```python
from build123d import *

# Parameters (mm, degrees)
SKIZZE2_W                        = 120
SKIZZE2_H                        = 39.364160046
AUFSATZ_LINEAR_AUSTRAGEN1_DEPTH  = 30
SKIZZE24_R                       = 1.55
SCHNITT_LINEAR_AUSTRAGEN4_DEPTH  = 130.805766806
SKIZZE46_R                       = 2.85
SCHNITT_LINEAR_AUSTRAGEN15_DEPTH = 10
SCHNITT_LINEAR_START             = -5
SCHNITT_LINEAR_AUSTRAGEN25_DEPTH = 2.7
LINEARES_MUSTER1_COUNT           = 5
LINEARES_MUSTER1_PITCH           = 20
SPIEGELN2_COPY_1_SKETCH_R        = 2.85
SPIEGELN2_COPY_1_DEPTH           = 10
SPIEGELN2_COPY_2_SKETCH_R        = 2.85
SPIEGELN2_COPY_2_DEPTH           = 10
SPIEGELN2_COPY_3_SKETCH_R        = 2.85
SPIEGELN2_COPY_3_DEPTH           = 10
SPIEGELN2_COPY_4_SKETCH_R        = 2.85
SPIEGELN2_COPY_4_DEPTH           = 10
SPIEGELN2_START                  = -5
SPIEGELN2_COPY_5_DEPTH           = 2.7
SPIEGELN2_COPY_6_DEPTH           = 2.7
SPIEGELN2_COPY_7_DEPTH           = 2.7
SPIEGELN2_COPY_8_DEPTH           = 2.7
SKIZZE51_R                       = 1.55
SCHNITT_LINEAR_AUSTRAGEN26_DEPTH = 130.805766806
SKIZZE67_R                       = 0.5
SCHNITT_LINEAR_AUSTRAGEN28_DEPTH = 16
SKIZZE68_R                       = 0.65
SCHNITT_LINEAR_AUSTRAGEN30_DEPTH = 16
SKIZZE70_R                       = 2
SCHNITT_LINEAR_AUSTRAGEN31_DEPTH = 6
ABSPALTEN3_START                 = 15
ABSPALTEN3_OUTLINE_W             = 120
ABSPALTEN3_OUTLINE_H             = 39.364160046
ABSPALTEN3_OUTLINE_R             = 1.55
ABSPALTEN3_DEPTH                 = 15


# Read off the part's stored shape, not the designer's step: Abspalten3
with BuildPart() as part:
    # Skizze2 → Aufsatz-Linear austragen1 (new body)
    with BuildSketch(Plane.XY):
        with Locations((60, 19.682080023)):
            Rectangle(SKIZZE2_W, SKIZZE2_H)
    extrude(amount=AUFSATZ_LINEAR_AUSTRAGEN1_DEPTH)

    # Skizze24 → Schnitt-Linear austragen4 (cut, through all)
    with BuildSketch(Plane.XY.offset(30)):
        with Locations((20, 31.364160046)):
            Circle(SKIZZE24_R)
        with Locations((40, 31.364160046)):
            Circle(SKIZZE24_R)
        with Locations((60, 31.364160046)):
            Circle(SKIZZE24_R)
        with Locations((80, 31.364160046)):
            Circle(SKIZZE24_R)
        with Locations((100, 31.364160046)):
            Circle(SKIZZE24_R)
    schnitt_linear_austragen4 = extrude(amount=-SCHNITT_LINEAR_AUSTRAGEN4_DEPTH, mode=Mode.SUBTRACT)

    # Skizze46 → Schnitt-Linear austragen15 (cut)
    with BuildSketch(Plane(origin=(0, 0, 0), x_dir=(-1, 0, 0), z_dir=(0, 0, -1))):
        with Locations((-100, 31.364160046)):
            Circle(SKIZZE46_R)
    schnitt_linear_austragen15 = extrude(amount=-SCHNITT_LINEAR_AUSTRAGEN15_DEPTH, mode=Mode.SUBTRACT)

    # Skizze50 → Schnitt-Linear austragen25 (cut)
    with BuildSketch(Plane.XY.offset(30).offset(SCHNITT_LINEAR_START)):
        Polygon((97.15, 33.009608314), (97.15, 39.364160046), (102.85, 39.364160046), (102.85, 33.009608314), (102.85, 29.718711779), (100, 28.073263512), (97.15, 29.718711779), align=None)
    schnitt_linear_austragen25 = extrude(amount=-SCHNITT_LINEAR_AUSTRAGEN25_DEPTH, mode=Mode.SUBTRACT)

    # Lineares Muster1: Schnitt-Linear austragen15, Schnitt-Linear austragen25 ×5
    with Locations(*[(-i * LINEARES_MUSTER1_PITCH, 0, 0) for i in range(1, LINEARES_MUSTER1_COUNT)]):
        add(schnitt_linear_austragen15, mode=Mode.SUBTRACT)
        add(schnitt_linear_austragen25, mode=Mode.SUBTRACT)

    # Spiegeln2: Schnitt-Linear austragen15, Schnitt-Linear austragen25 across plane
    add(schnitt_linear_austragen15.mirror(Plane.ZX.offset(19.764160046)), mode=Mode.SUBTRACT)
    add(schnitt_linear_austragen25.mirror(Plane.ZX.offset(19.764160046)), mode=Mode.SUBTRACT)

    # Spiegeln2 copy 1 sketch → Spiegeln2 copy 1 (cut)
    with BuildSketch(Plane(origin=(-20, 39.528320093, 0), x_dir=(-1, 0, 0), z_dir=(0, 0, -1))):
        with Locations((-100, -31.364160046)):
            Circle(SPIEGELN2_COPY_1_SKETCH_R)
    extrude(amount=-SPIEGELN2_COPY_1_DEPTH, mode=Mode.SUBTRACT)

    # Spiegeln2 copy 2 sketch → Spiegeln2 copy 2 (cut)
    with BuildSketch(Plane(origin=(-40, 39.528320093, 0), x_dir=(-1, 0, 0), z_dir=(0, 0, -1))):
        with Locations((-100, -31.364160046)):
            Circle(SPIEGELN2_COPY_2_SKETCH_R)
    extrude(amount=-SPIEGELN2_COPY_2_DEPTH, mode=Mode.SUBTRACT)

    # Spiegeln2 copy 3 sketch → Spiegeln2 copy 3 (cut)
    with BuildSketch(Plane(origin=(-60, 39.528320093, 0), x_dir=(-1, 0, 0), z_dir=(0, 0, -1))):
        with Locations((-100, -31.364160046)):
            Circle(SPIEGELN2_COPY_3_SKETCH_R)
    extrude(amount=-SPIEGELN2_COPY_3_DEPTH, mode=Mode.SUBTRACT)

    # Spiegeln2 copy 4 sketch → Spiegeln2 copy 4 (cut)
    with BuildSketch(Plane(origin=(-80, 39.528320093, 0), x_dir=(-1, 0, 0), z_dir=(0, 0, -1))):
        with Locations((-100, -31.364160046)):
            Circle(SPIEGELN2_COPY_4_SKETCH_R)
    extrude(amount=-SPIEGELN2_COPY_4_DEPTH, mode=Mode.SUBTRACT)

    # Spiegeln2 copy 5 sketch → Spiegeln2 copy 5 (cut)
    with BuildSketch(Plane(origin=(-20, 39.528320093, 30), x_dir=(1, 0, 0), z_dir=(0, 0, 1)).offset(SPIEGELN2_START)):
        Polygon((97.15, -33.009608314), (97.15, -39.364160046), (102.85, -39.364160046), (102.85, -33.009608314), (102.85, -29.718711779), (100, -28.073263512), (97.15, -29.718711779), align=None)
    extrude(amount=-SPIEGELN2_COPY_5_DEPTH, mode=Mode.SUBTRACT)

    # Spiegeln2 copy 6 sketch → Spiegeln2 copy 6 (cut)
    with BuildSketch(Plane(origin=(-40, 39.528320093, 30), x_dir=(1, 0, 0), z_dir=(0, 0, 1)).offset(SPIEGELN2_START)):
        Polygon((97.15, -33.009608314), (97.15, -39.364160046), (102.85, -39.364160046), (102.85, -33.009608314), (102.85, -29.718711779), (100, -28.073263512), (97.15, -29.718711779), align=None)
    extrude(amount=-SPIEGELN2_COPY_6_DEPTH, mode=Mode.SUBTRACT)

    # Spiegeln2 copy 7 sketch → Spiegeln2 copy 7 (cut)
    with BuildSketch(Plane(origin=(-60, 39.528320093, 30), x_dir=(1, 0, 0), z_dir=(0, 0, 1)).offset(SPIEGELN2_START)):
        Polygon((97.15, -33.009608314), (97.15, -39.364160046), (102.85, -39.364160046), (102.85, -33.009608314), (102.85, -29.718711779), (100, -28.073263512), (97.15, -29.718711779), align=None)
    extrude(amount=-SPIEGELN2_COPY_7_DEPTH, mode=Mode.SUBTRACT)

    # Spiegeln2 copy 8 sketch → Spiegeln2 copy 8 (cut)
    with BuildSketch(Plane(origin=(-80, 39.528320093, 30), x_dir=(1, 0, 0), z_dir=(0, 0, 1)).offset(SPIEGELN2_START)):
        Polygon((97.15, -33.009608314), (97.15, -39.364160046), (102.85, -39.364160046), (102.85, -33.009608314), (102.85, -29.718711779), (100, -28.073263512), (97.15, -29.718711779), align=None)
    extrude(amount=-SPIEGELN2_COPY_8_DEPTH, mode=Mode.SUBTRACT)

    # Spiegeln3: Schnitt-Linear austragen4 across plane
    add(schnitt_linear_austragen4.mirror(Plane.ZX.offset(19.764160046)), mode=Mode.SUBTRACT)

    # Skizze51 → Schnitt-Linear austragen26 (cut, through all)
    with BuildSketch(Plane.XY.offset(30)):
        with Locations((5, 34.364160046)):
            Circle(SKIZZE51_R)
        with Locations((115, 5)):
            Circle(SKIZZE51_R)
    extrude(amount=-SCHNITT_LINEAR_AUSTRAGEN26_DEPTH, mode=Mode.SUBTRACT)

    # Skizze66 → Schnitt-Rotation5 (revolve, cut)
    with BuildSketch(Plane.XY.offset(15), mode=Mode.PRIVATE) as schnitt_rotation5_sk:
        Polygon((110, 19.682080023), (110, 21.182080023), (10, 22.682080023), (10, 19.682080023), align=None)
        Polygon((105, 19.682080023), (105, 23.757361257), (15, 25.107361257), (15, 19.682080023), align=None)
    revolve(schnitt_rotation5_sk.sketch.rotate(Axis((10, 19.682080023, 15), (1, 0, 0)), 180), axis=Axis((10, 19.682080023, 15), (1, 0, 0)), mode=Mode.SUBTRACT)

    # Skizze67 → Schnitt-Linear austragen28 (cut)
    with BuildSketch(Plane(origin=(120, 0, 0), x_dir=(0, 0, -1), z_dir=(1, 0, 0))):
        with Locations((-18.5, 19.764160046)):
            Circle(SKIZZE67_R)
    schnitt_linear_austragen28 = extrude(amount=-SCHNITT_LINEAR_AUSTRAGEN28_DEPTH, mode=Mode.SUBTRACT)

    # Spiegeln5: Schnitt-Linear austragen28 across plane
    add(schnitt_linear_austragen28.mirror(Plane.XY.offset(15)), mode=Mode.SUBTRACT)

    # Skizze68 → Schnitt-Linear austragen30 (cut)
    with BuildSketch(Plane.ZY):
        with Locations((10.25, 19.764160046)):
            Circle(SKIZZE68_R)
    extrude(amount=-SCHNITT_LINEAR_AUSTRAGEN30_DEPTH, mode=Mode.SUBTRACT)

    # Skizze70 → Schnitt-Linear austragen31 (cut)
    with BuildSketch(Plane.ZY):
        with Locations((10.25, 19.764160046)):
            Circle(SKIZZE70_R)
    extrude(amount=-SCHNITT_LINEAR_AUSTRAGEN31_DEPTH, mode=Mode.SUBTRACT)

    # Abspalten3 outline → Abspalten3 (cut)
    with BuildSketch(Plane.XY.offset(ABSPALTEN3_START)):
        with Locations((60, 19.682080023)):
            Rectangle(ABSPALTEN3_OUTLINE_W, ABSPALTEN3_OUTLINE_H)
        with Locations((115, 5)):
            Circle(ABSPALTEN3_OUTLINE_R, mode=Mode.SUBTRACT)
        with Locations((5, 34.364160046)):
            Circle(ABSPALTEN3_OUTLINE_R, mode=Mode.SUBTRACT)
        with Locations((20, 31.364160046)):
            Circle(ABSPALTEN3_OUTLINE_R, mode=Mode.SUBTRACT)
        with Locations((40, 31.364160046)):
            Circle(ABSPALTEN3_OUTLINE_R, mode=Mode.SUBTRACT)
        with Locations((60, 31.364160046)):
            Circle(ABSPALTEN3_OUTLINE_R, mode=Mode.SUBTRACT)
        with Locations((80, 31.364160046)):
            Circle(ABSPALTEN3_OUTLINE_R, mode=Mode.SUBTRACT)
        with Locations((100, 31.364160046)):
            Circle(ABSPALTEN3_OUTLINE_R, mode=Mode.SUBTRACT)
        with Locations((20, 8.164160046)):
            Circle(ABSPALTEN3_OUTLINE_R, mode=Mode.SUBTRACT)
        with Locations((40, 8.164160046)):
            Circle(ABSPALTEN3_OUTLINE_R, mode=Mode.SUBTRACT)
        with Locations((60, 8.164160046)):
            Circle(ABSPALTEN3_OUTLINE_R, mode=Mode.SUBTRACT)
        with Locations((80, 8.164160046)):
            Circle(ABSPALTEN3_OUTLINE_R, mode=Mode.SUBTRACT)
        with Locations((100, 8.164160046)):
            Circle(ABSPALTEN3_OUTLINE_R, mode=Mode.SUBTRACT)
    extrude(amount=ABSPALTEN3_DEPTH, mode=Mode.SUBTRACT)


solid = part.part
```
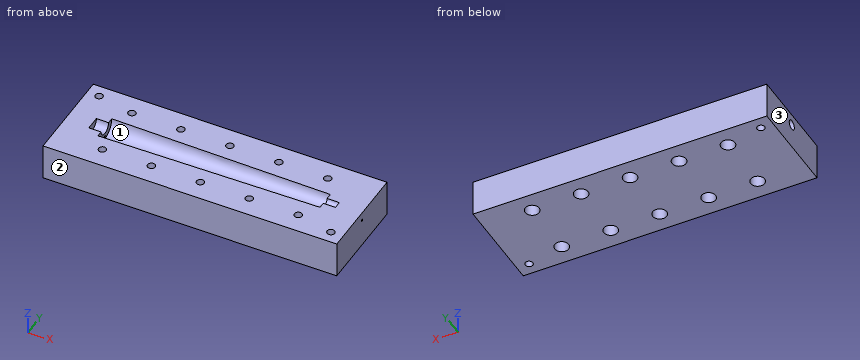
Geometry check sheet. Reference: the model listing, model coordinates, mm. Face numbers are marked on the shaded views. Give positions to 0.01 mm unless a question says otherwise; leave off trailing zeros. Write each loop counter-clockwise with the first axis right and the second up, starting at its lowest first coordinate (ties: lowest second). Pieces come first, ordered by that corner, then holes. Notation, with made-up numbers: (38, 15) - (63, 15) arc R13 cw to (63, 33) - close; hole circle Ø11 at (46.25, -2.75). An arc over 180 degrees is marked (long way). Use a Markdown table: item, result.
Q1. Section check B-B, the plane x = 20. Enter the section's corners in (y, z), then the cut area to 3 significant figures.
Computed:
| item | result |
|---|---|
| outline | (0, 0) - (5.31, 0) - (5.31, 10) - (6.61, 10) - (6.61, 15) - (0, 15) - close; (9.71, 10) - (11.01, 10) - (11.01, 0) - (28.51, 0) - (28.51, 10) - (29.81, 10) - (29.81, 15) - (25.03, 15) arc R5.35 cw to (14.33, 15) - (9.71, 15) - close; (32.91, 10) - (34.21, 10) - (34.21, 0) - (39.36, 0) - (39.36, 15) - (32.91, 15) - close |
| area | 400 mm² |
Q2. Section check D-D, the plane x = 100. Enter the section's corners in (y, z).
Computed:
| item | result |
|---|---|
| outline | (0, 0) - (5.31, 0) - (5.31, 10) - (6.61, 10) - (6.61, 15) - (0, 15) - close; (9.71, 10) - (11.01, 10) - (11.01, 0) - (28.51, 0) - (28.51, 10) - (29.81, 10) - (29.81, 15) - (23.83, 15) arc R4.15 cw to (15.53, 15) - (9.71, 15) - close; (32.91, 10) - (34.21, 10) - (34.21, 0) - (39.36, 0) - (39.36, 15) - (32.91, 15) - close |
Q3. Section check C-C, the plane z = 6. Give the number of separate pieces and of enclosed holes in the cut face, then the cut area to 3 significant figures.
Computed:
| item | result |
|---|---|
| separate pieces | 1 |
| enclosed holes | 12 |
| area | 4,450 mm² |
Q4. Thickness scan on L1, parallel to Y at x = 60, z = 6.75; L2, parallel to X at y = 31, z = 8.5; L3, parallel to Y at x = 2.55, z = 10.25. Record the ranges inside material, lowest first. Write a range as [from, to].
Computed:
| item | result |
|---|---|
| L1 | y = [0, 5.31], [11.01, 28.51], [34.21, 39.36] |
| L2 | x = [0, 17.17], [22.83, 37.17], [42.83, 57.17], [62.83, 77.17], [82.83, 97.17], [102.83, 120] |
| L3 | y = [0, 17.76], [21.76, 39.36] |
Q5. Go/stop test with a flat-tipped pin: P1, Ø3.5, axis at x = 20, y = 8.16, coming from the -Z side. Record where the tip stops, or that it passes through.
Computed:
| item | result |
|---|---|
| P1 | stops at z = 10 |
Q6. Section check A-A, the plane x = 115. Enter the section's corners in (y, z), then the cut area to 3 significant figures.
Computed:
| item | result |
|---|---|
| outline | (0, 0) - (3.45, 0) - (3.45, 15) - (0, 15) - close; (6.55, 0) - (39.36, 0) - (39.36, 15) - (6.55, 15) - close; hole circle Ø1 at (19.76, 11.5) |
| area | 543 mm² |
Q7. Draft check along Y on the marked faces 1, 2 and 3. Enter one of: pulls with the +Y half, pulls with the -Y half, needs draft (parallel to the pull), parting line crosses it, or undercut.
Computed:
| item | result |
|---|---|
| face 1 | undercut |
| face 2 | pulls with the -Y half |
| face 3 | needs draft |
